Read the model definition and answer for the solid it produces. Units are mm, in the model's axes. Face numbers are marked on the shaded views. A direction names the side the tool comes from. Coordinates: 2 decimals unless noted, no trailing zeros. Write each loop counter-clockwise with the first axis right and the second up, starting at its lowest first coordinate (ties: lowest second). Pieces come first, ordered by that corner, then holes.
1) The part is cut by section D-D (y = 5). Determine the outline of the cut face in (x, z).
2) Which of the six approach directions +Z, -Z, +X, -X, +Y, -Y give full straight-line access (tool end or side, diameter ignored) to the marked faces 1 and 2?
3) Determine the mould class of the marked faces 3, 4, 5 and 6 for opening direction X: +X half, -X half, draft (parallel to the pull), parting line (faces both ways), or undercut.
4) The part is cut by section A-A (y = -0.5). Determine the outline of the cut face in (x, z), then the cut area to 3 significant figures.
5) The part is cut by section B-B (z = -20). Determine the outline of the cut face in (x, y).
6) Each of these flat-tipped pins is pushed along its axis until it touches: pin 1 Ø10 at (x, z) = (7.5, -16.5) entering from -Y; pin 2 Ø16 at (y, z) = (-1, -38) entering from -X; pin 3 Ø1 at (x, z) = (13, -13.5) entering from +Y. Where does it stop, or does it pass through?
7) Find the intervals of material crossed by line 1 (X direction, y = -1.5, z = -6); line 2 (Y direction, x = 22, z = -24); line 3 (Z direction, x = -11.5, y = 9.5), in increasing order.
8) The part is cut by section C-C (z = -14). Determine the outline of the cut face in (x, y), then the cut area to 3 significant figures.
from build123d import *

# Parameters (mm, degrees)
F0_R     = 1.45
F1_DEPTH = 17
F2_DEPTH = 51
F3_R     = 1
F4_DEPTH = 42.6430173342
F3_R_2   = 2.4
F5_DEPTH = 4
F6_SIZE  = 2


with BuildPart() as f1:
    # F0 (on Top) → F1 (new body)
    with BuildSketch(Plane.XY):
        with BuildLine():
            ThreePointArc((-6.2514946472, 3.0411327703), (-8.8875336165, 9.4050938009), (-6.2514946472, 15.7690548316))
            Line((-6.2514946472, 15.7690548316), (-29.9395718169, 39.4571320014))
            Line((-29.9395718169, 39.4571320014), (-36.3035328476, 33.0931709707))
            Line((-36.3035328476, 33.0931709707), (-6.2514946472, 3.0411327703))
        make_face()
        with Locations((-29.0556883405, 32.2092874942)):
            Circle(F0_R, mode=Mode.SUBTRACT)
        with BuildLine():
            Line((-6.2514946472, 3.0411327703), (0.1124663835, 9.4050938009))
            Line((0.1124663835, 9.4050938009), (-6.2514946472, 15.7690548316))
            ThreePointArc((-6.2514946472, 15.7690548316), (-8.8875336165, 9.4050938009), (-6.2514946472, 3.0411327703))
        make_face()
        with Locations((-7.1353781237, 10.2889772774)):
            Circle(F0_R, mode=Mode.SUBTRACT)
        with BuildLine():
            Line((0.1124663835, 0.4050938009), (0.1124663835, 9.4050938009))
            Line((0.1124663835, 9.4050938009), (-6.2514946472, 3.0411327703))
            ThreePointArc((-6.2514946472, 3.0411327703), (-3.3316845078, 1.0901780083), (0.1124663835, 0.4050938009))
        make_face()
        with BuildLine():
            Line((9.1124663835, 9.4050938009), (0.1124663835, 9.4050938009))
            Line((0.1124663835, 9.4050938009), (0.1124663835, 0.4050938009))
            ThreePointArc((0.1124663835, 0.4050938009), (1.1187766024, 0.4615296488), (2.1124663835, 0.6301294135))
            Line((2.1124663835, 0.6301294135), (2.1124663835, 7.4050938009))
            Line((2.1124663835, 7.4050938009), (8.8874307709, 7.4050938009))
            ThreePointArc((8.8874307709, 7.4050938009), (9.0560305356, 8.398783582), (9.1124663835, 9.4050938009))
        make_face()
        with BuildLine():
            ThreePointArc((2.1124663835, 0.6301294135), (1.1187766024, 0.4615296488), (0.1124663835, 0.4050938009))
            Line((0.1124663835, 0.4050938009), (0.1124663835, -12.5949061991))
            Line((0.1124663835, -12.5949061991), (2.1124663835, -12.5949061991))
            Line((2.1124663835, -12.5949061991), (2.1124663835, 0.6301294135))
        make_face()
        with BuildLine():
            Line((24.1124663835, 9.4050938009), (9.1124663835, 9.4050938009))
            ThreePointArc((9.1124663835, 9.4050938009), (9.0560305356, 8.398783582), (8.8874307709, 7.4050938009))
            Line((8.8874307709, 7.4050938009), (22.1124663835, 7.4050938009))
            Line((22.1124663835, 7.4050938009), (22.1124663835, -12.5949061991))
            Line((22.1124663835, -12.5949061991), (21.1124663835, -12.5949061991))
            Line((21.1124663835, -12.5949061991), (21.1124663835, -14.483826209))
            Line((21.1124663835, -14.483826209), (24.1124663835, -14.483826209))
            Line((24.1124663835, -14.483826209), (24.1124663835, -12.5945746742))
            Line((24.1124663835, -12.5945746742), (24.1124663835, 9.4050938009))
        make_face()
    extrude(amount=-F1_DEPTH)

    # F0 (on Top) → F2 (join)
    with BuildSketch(Plane.XY):
        with BuildLine():
            ThreePointArc((2.1124663835, 0.6301294135), (1.1187766024, 0.4615296488), (0.1124663835, 0.4050938009))
            Line((0.1124663835, 0.4050938009), (0.1124663835, -12.5949061991))
            Line((0.1124663835, -12.5949061991), (2.1124663835, -12.5949061991))
            Line((2.1124663835, -12.5949061991), (2.1124663835, 0.6301294135))
        make_face()
        with BuildLine():
            Line((9.1124663835, 9.4050938009), (0.1124663835, 9.4050938009))
            Line((0.1124663835, 9.4050938009), (0.1124663835, 0.4050938009))
            ThreePointArc((0.1124663835, 0.4050938009), (1.1187766024, 0.4615296488), (2.1124663835, 0.6301294135))
            Line((2.1124663835, 0.6301294135), (2.1124663835, 7.4050938009))
            Line((2.1124663835, 7.4050938009), (8.8874307709, 7.4050938009))
            ThreePointArc((8.8874307709, 7.4050938009), (9.0560305356, 8.398783582), (9.1124663835, 9.4050938009))
        make_face()
        with BuildLine():
            Line((24.1124663835, 9.4050938009), (9.1124663835, 9.4050938009))
            ThreePointArc((9.1124663835, 9.4050938009), (9.0560305356, 8.398783582), (8.8874307709, 7.4050938009))
            Line((8.8874307709, 7.4050938009), (22.1124663835, 7.4050938009))
            Line((22.1124663835, 7.4050938009), (22.1124663835, -12.5949061991))
            Line((22.1124663835, -12.5949061991), (21.1124663835, -12.5949061991))
            Line((21.1124663835, -12.5949061991), (21.1124663835, -14.483826209))
            Line((21.1124663835, -14.483826209), (24.1124663835, -14.483826209))
            Line((24.1124663835, -14.483826209), (24.1124663835, -12.5945746742))
            Line((24.1124663835, -12.5945746742), (24.1124663835, 9.4050938009))
        make_face()
    extrude(amount=-F2_DEPTH)

    # F3 (on face) → F4 (cut, through all)
    with BuildSketch(Plane(origin=(4.7587800922, 4.7587800922, 0), x_dir=(-0.7071067812, 0.7071067812, 0), z_dir=(0.7071067812, 0.7071067812, 0))):
        with Locations((23.0708798619, -8)):
            Circle(F3_R)
    extrude(amount=-F4_DEPTH, mode=Mode.SUBTRACT)

    # F3 (on face) → F5 (cut)
    with BuildSketch(Plane(origin=(4.7587800922, 4.7587800922, 0), x_dir=(-0.7071067812, 0.7071067812, 0), z_dir=(0.7071067812, 0.7071067812, 0))):
        with Locations((23.0708798619, -8)):
            Circle(F3_R_2)
        with Locations((23.0708798619, -8)):
            Circle(F3_R, mode=Mode.SUBTRACT)
    extrude(amount=-F5_DEPTH, mode=Mode.SUBTRACT)

    # F6
    f6_edges = [f1.edges().sort_by_distance(p)[0] for p in [
        (-17.21165, 14.001288, -8),
    ]]
    chamfer(f6_edges, length=F6_SIZE)


solid = f1.part
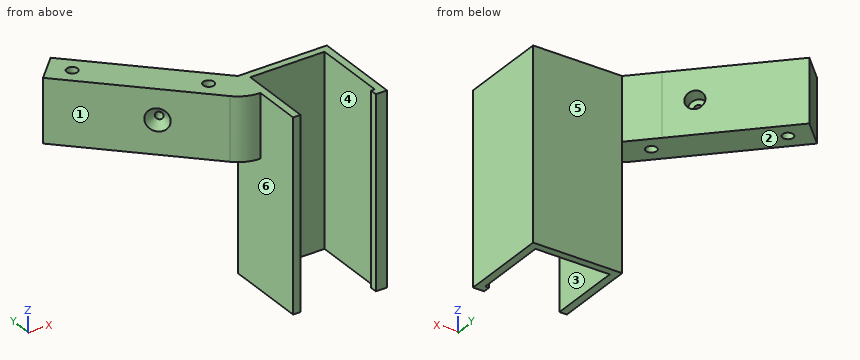
Reported:
1. outline: (-8.21, -17) - (0.11, -17) - (0.11, -51) - (2.11, -51) - (2.11, 0) - (-8.21, 0) - close; (22.11, -51) - (24.11, -51) - (24.11, 0) - (22.11, 0) - close
2. face 1: +Z, -Z, -X, -Y
2. face 2: -Z, -X, +Y, -Y
3. face 3: undercut
3. face 4: undercut
3. face 5: draft
3. face 6: -X half
4. outline: (0.11, -51) - (2.11, -51) - (2.11, 0) - (0.11, 0) - close; (22.11, -51) - (24.11, -51) - (24.11, 0) - (22.11, 0) - close
4. area: 204 mm2
5. outline: (0.11, -12.59) - (2.11, -12.59) - (2.11, 7.41) - (22.11, 7.41) - (22.11, -12.59) - (21.11, -12.59) - (21.11, -14.48) - (24.11, -14.48) - (24.11, 9.41) - (0.11, 9.41) - close
6. pin 1: stops at y = 7.41
6. pin 2: stops at x = 0.11
6. pin 3: stops at y = 9.41
7. line 1: x = 0.11 to 2.11, 22.11 to 24.11
7. line 2: y = -14.48 to -12.59, 7.41 to 9.41
7. line 3: z = -17 to 0
8. outline: (-36.3, 33.09) - (-6.25, 3.04) arc R9 ccw to (0.11, 0.41) - (0.11, -12.59) - (2.11, -12.59) - (2.11, 7.41) - (22.11, 7.41) - (22.11, -12.59) - (21.11, -12.59) - (21.11, -14.48) - (24.11, -14.48) - (24.11, 9.41) - (0.11, 9.41) - (-29.94, 39.46) - close; hole circle Ø2.9 at (-29.06, 32.21); hole circle Ø2.9 at (-7.14, 10.29)
8. area: 535 mm2
